Check sheet for the modelled part. Datum: model origin and axes. Units: mm. Coordinates: 2 decimals unless noted, no trailing zeros. Loops run counter-clockwise (first coordinate to the right, second up) from the corner with the lowest first, then second, coordinate; pieces in that order, holes last. Notation, with made-up numbers: (82, 73) - (87, 73) arc R27 ccw to (87, 109) - close; hole circle Ø10 at (66.25, 26). An arc over 180 degrees is marked (long way). Use a Markdown table: item, result. Add a question column.
1) Sectioned sample at B-B, the plane x = -92. Enter the section's corners in (y, z).
2) Sectioned sample at A-A, the plane y = -3.5. Enter the section's corners in (x, z).
3) Sectioned sample at C-C, the plane z = 154. Enter the section's corners in (x, y).
4) Thickness scan on line 1 (X direction, y = -3.25, z = 130); line 2 (X direction, y = -3.75, z = 133); line 3 (Z direction, x = -106, y = -5.5). Record the ranges inside material, lowest first.
from build123d import *

# Parameters (mm, degrees)
F0_W     = 152.4
F0_H     = 152.4
F1_DEPTH = 6.35
F3_DEPTH = 25.4
F5_DEPTH = 25.4


with BuildPart() as f1:
    # F0 (on Front) → F1 (new body)
    with BuildSketch(Plane.XZ):
        with Locations((-99.789874, 97.348559)):
            Rectangle(F0_W, F0_H)
    extrude(amount=F1_DEPTH)

    # F2 (on face) → F3 (cut)
    with BuildSketch(Plane.XZ.offset(6.35)):
        Polygon((-163.289874, 173.548559), (-175.989874, 173.548559), (-175.989874, 148.148559), align=None)
        Polygon((-23.589874, 173.548559), (-36.289874, 173.548559), (-23.589874, 148.148559), align=None)
    extrude(amount=-F3_DEPTH, mode=Mode.SUBTRACT)

    # F4 (on face) → F5 (cut)
    with BuildSketch(Plane.XZ.offset(6.35)):
        with BuildLine():
            ThreePointArc((-87.089874, 122.748559), (-90.809618, 131.728815), (-99.789874, 135.448559))
            ThreePointArc((-99.789874, 135.448559), (-108.77013, 113.768303), (-87.089874, 122.748559))
        make_face()
    extrude(amount=-F5_DEPTH, mode=Mode.SUBTRACT)


solid = f1.part
Solved:
| question | item | result |
|---|---|---|
| 1 | outline | (-6.35, 21.15) - (0, 21.15) - (0, 112.72) - (-6.35, 112.72) - close; (-6.35, 132.78) - (0, 132.78) - (0, 173.55) - (-6.35, 173.55) - close |
| 2 | outline | (-175.99, 21.15) - (-23.59, 21.15) - (-23.59, 148.15) - (-36.29, 173.55) - (-163.29, 173.55) - (-175.99, 148.15) - close; hole circle Ø25.4 at (-99.79, 122.75) |
| 3 | outline | (-173.06, -6.35) - (-26.52, -6.35) - (-26.52, 0) - (-173.06, 0) - close |
| 4 | line 1 | x = -175.99 to -110.22, -89.36 to -23.59 |
| 4 | line 2 | x = -175.99 to -107.29, -92.29 to -23.59 |
| 4 | line 3 | z = 21.15 to 111.67, 133.83 to 173.55 |
